```python
from build123d import *

# Parameters (mm, degrees)
F0_R      = 60
F1_DEPTH  = 20
F3_DEPTH  = 10
F4_W      = 5
F4_H      = 70
F5_DEPTH  = 60
F7_DEPTH  = 3
F8_W      = 3.5498722099
F8_H      = 4.546627143
F9_DEPTH  = 6
F10_W     = 10
F10_H     = 8
F11_DEPTH = 20.001


with BuildPart() as f1:
    # F0 (on Front) → F1 (new body)
    with BuildSketch(Plane.XZ):
        Circle(F0_R)
    extrude(amount=F1_DEPTH)

    # F2 (on face) → F3 (cut)
    with BuildSketch(Plane.XZ.offset(20)):
        with BuildLine():
            Line((-25, -12.5), (-25, 12.5))
            Line((-25, 12.5), (-58.6834729715, 12.5))
            ThreePointArc((-58.6834729715, 12.5), (-59.6699605258, 6.2845692656), (-60, 0))
            ThreePointArc((-60, 0), (-59.6699605258, -6.2845692656), (-58.6834729715, -12.5))
            Line((-58.6834729715, -12.5), (-25, -12.5))
        make_face()
        with BuildLine():
            Line((58.6834729715, 12.5), (25, 12.5))
            Line((25, 12.5), (25, -12.5))
            Line((25, -12.5), (58.6834729715, -12.5))
            ThreePointArc((58.6834729715, -12.5), (59.6699605258, -6.2845692656), (60, 0))
            ThreePointArc((60, 0), (59.6699605258, 6.2845692656), (58.6834729715, 12.5))
        make_face()
    extrude(amount=-F3_DEPTH, mode=Mode.SUBTRACT)

    # F4 (on Right) → F5 (cut, symmetric)
    with BuildSketch(Plane.YZ):
        with Locations((-12.5, 0)):
            Rectangle(F4_W, F4_H)
    extrude(amount=F5_DEPTH, both=True, mode=Mode.SUBTRACT)

    # F6 (on face) → F7 (cut)
    with BuildSketch(Plane.XZ.offset(10)):
        with BuildLine():
            Line((30, -22.5), (30, -25))
            Line((30, -25), (-30, -25))
            Line((-30, -25), (-30, -22.5))
            Line((-30, -22.5), (-55.6214886532, -22.5))
            ThreePointArc((-55.6214886532, -22.5), (-54.531492065, -25.0263136152), (-53.3268225193, -27.5))
            Line((-53.3268225193, -27.5), (0, -27.5))
            Line((0, -27.5), (53.3268225193, -27.5))
            ThreePointArc((53.3268225193, -27.5), (54.531492065, -25.0263136152), (55.6214886532, -22.5))
            Line((55.6214886532, -22.5), (30, -22.5))
        make_face()
        with BuildLine():
            Line((30, 25), (30, 22.5))
            Line((30, 22.5), (55.6214886532, 22.5))
            ThreePointArc((55.6214886532, 22.5), (54.531492065, 25.0263136152), (53.3268225193, 27.5))
            Line((53.3268225193, 27.5), (0, 27.5))
            Line((0, 27.5), (-53.3268225193, 27.5))
            ThreePointArc((-53.3268225193, 27.5), (-54.531492065, 25.0263136152), (-55.6214886532, 22.5))
            Line((-55.6214886532, 22.5), (-30, 22.5))
            Line((-30, 22.5), (-30, 25))
            Line((-30, 25), (30, 25))
        make_face()
        Polygon((0, 22.5), (30, 22.5), (30, 25), (-30, 25), (-30, 22.5), align=None)
        Polygon((-30, -25), (30, -25), (30, -22.5), (0, -22.5), (-30, -22.5), align=None)
    extrude(amount=-F7_DEPTH, mode=Mode.SUBTRACT)

    # F8 (on face) → F9 (join)
    with BuildSketch(Plane.XZ.offset(20)):
        Polygon((-5.9, -16.6), (-5.9, 5.9), (-10.2642504498, 5.9), (-10.2642504498, -21.146627143), (-2.3501277901, -21.146627143), (-2.3501277901, -16.6), align=None)
        Polygon((-10.2642504498, 5.9), (-5.9, 5.9), (5.9, 5.9), (5.9, -16.6), (5.9, -21.146627143), (9.9355150014, -21.146627143), (9.9355150014, 10.4155028239), (-10.2642504498, 10.4155028239), align=None)
        with Locations((4.1250638951, -18.8733135715)):
            Rectangle(F8_W, F8_H)
    extrude(amount=F9_DEPTH)

    # F10 (on face) → F11 (cut, through all)
    with BuildSketch(Plane.XZ.offset(20)):
        with Locations((0, -46.5785360177)):
            Rectangle(F10_W, F10_H)
    extrude(amount=-F11_DEPTH, mode=Mode.SUBTRACT)


solid = f1.part
```
The listing builds one solid part. Answer for the finished solid, in the listing's coordinates (mm). A direction names the side the tool comes from. Round coordinates to 2 decimals unless told otherwise and drop trailing zeros. Order: outer loops, then holes, each group sorted by start corner. A loop starts at its lowest first (then second) coordinate and runs counter-clockwise, first axis right, second up. Notation, with made-up numbers: (-15, 35.25) -> (18, 35.25) arc R9 ccw to (18, 50.25) -> close; hole circle Ø9 at (25.5, -6). An arc over 180 degrees is marked (long way). Answer as CSV lines item,"result".
Q1. A cutting plane is placed at C-C on z = 0. Determine the outline of the cut face in (x, y), plus the area to 3 significant figures.
Computed values:
outline,"(-60, -10) -> (60, -10) -> (60, 0) -> (-60, 0) -> close; (-25, -20) -> (-10.26, -20) -> (-10.26, -26) -> (-5.9, -26) -> (-5.9, -20) -> (5.9, -20) -> (5.9, -26) -> (9.94, -26) -> (9.94, -20) -> (25, -20) -> (25, -15) -> (-25, -15) -> close"
area,"1,500 mm^2"
Q2. Which of the six approach directions +Z, -Z, +X, -X, +Y, -Y give full straight-line access (tool end or side, diameter ignored) to faces 5 (the flat face through (1, -13, -35)), 6 (the flat face through (0, -23, 5.9)), 7 (the flat face through (42, -18, -12.5)), 8 (the flat face through (-25, -18, 0)), 9 (the flat face through (-6, -23, -21.147))?
Computed values:
face 5,"+X, -X"
face 6,"-Y"
face 7,"+X, -Y"
face 8,"-X, -Y"
face 9,"-Z, +X, -X, -Y"
Q3. A cutting plane is placed at A-A on x = 0. Determine the outline of the cut face in (y, z), plus the area to 3 significant figures.
Computed values:
outline,"(-26, 5.9) -> (-20, 5.9) -> (-20, -42.58) -> (0, -42.58) -> (0, 60) -> (-20, 60) -> (-20, 10.42) -> (-26, 10.42) -> close; (-20, -60) -> (0, -60) -> (0, -50.58) -> (-20, -50.58) -> close; hole (-15, -35) -> (-10, -35) -> (-10, -27.5) -> (-7, -27.5) -> (-7, -22.5) -> (-10, -22.5) -> (-10, 22.5) -> (-7, 22.5) -> (-7, 27.5) -> (-10, 27.5) -> (-10, 35) -> (-15, 35) -> close"
area,"1,890 mm^2"
Q4. For a pull along X with two mould halves and no side action, classify faces 1 (the cylindrical face through (-44.222, -9.86, 40.551)), 2 (the flat face through (-1, -10, 31)), 3 (the flat face through (-10.264, -23, -5)), 4 (the flat face through (2.35, -23, -19)) as +X half, -X half, draft (parallel to the pull), parting line (faces both ways), or undercut.
Computed values:
face 1,"parting line"
face 2,"draft"
face 3,"-X half"
face 4,"undercut"
Q5. A cutting plane is placed at B-B on y = -12. Determine the outline of the cut face in (x, z).
Computed values:
outline,"(-48.73, -35) arc R60 ccw to (48.73, -35) -> close; (-48.73, 35) -> (48.73, 35) arc R60 ccw to start; hole (-5, -50.58) -> (5, -50.58) -> (5, -42.58) -> (-5, -42.58) -> close"
Q6. Given pin 1 (5 mm diameter, centred on y = -23.5, z = -6, fed in from +X); pin 2 (1.8 mm diameter, centred on x = 7.5, y = -23.5, fed in from -Z); pin 3 (2.5 mm diameter, centred on x = 7.5, z = 24.5, fed in from -Y); pin 4 (12 mm diameter, centred on x = 8, z = 40, fed in from +Y), each flat-ended and moving along its own axis, determine where each tip first touches the part or whether it passes through.
Computed values:
pin 1,"stops at x = 9.94"
pin 2,"stops at z = -21.15"
pin 3,"stops at y = -20"
pin 4,"stops at y = 0"
Q7. A cutting plane is placed at D-D on y = -5.25. Determine the outline of the cut face in (x, z), plus the area to 3 significant figures.
Computed values:
outline,"circle Ø120 at (0, 0); hole (-5, -50.58) -> (5, -50.58) -> (5, -42.58) -> (-5, -42.58) -> close"
area,"11,200 mm^2"
Q8. Consider line 1 (Y direction, x = -16.5, z = -13); line 2 (Y direction, x = -4, z = 25); line 3 (Z direction, x = -30, y = -9.5). Determine where each line is inside the solid, lowest interval first. Write a range as from..to.
Computed values:
line 1,"y = -20..-15, -10..0"
line 2,"y = -20..-15, -7..0"
line 3,"z = -51.96..-27.5, -22.5..22.5, 27.5..51.96"
